from build123d import *

# Parameters (mm, degrees)
SKETCH1_R           = 2.54
BOSS_EXTRUDE1_DEPTH = 3.175
FILLET1_R           = 6.35
FILLET2_R           = 3.175


with BuildPart() as part:
    # Sketch1 → Boss-Extrude1 (new body)
    with BuildSketch(Plane(origin=(0, 0, 0), x_dir=(1, 0, 0), z_dir=(0, 1, 0))):
        Polygon((0, 0), (0, 88.9), (25.4, 88.9), (88.9, 25.4), (88.9, 0), align=None)
        with Locations(Location((12.7, 12.7, 0), (0, 0, 270))):
            Circle(SKETCH1_R, mode=Mode.SUBTRACT)
        with Locations(Location((25.4, 12.7, 0), (0, 0, 270))):
            Circle(SKETCH1_R, mode=Mode.SUBTRACT)
        with Locations(Location((38.1, 12.7, 0), (0, 0, 270))):
            Circle(SKETCH1_R, mode=Mode.SUBTRACT)
        with Locations(Location((50.8, 12.7, 0), (0, 0, 270))):
            Circle(SKETCH1_R, mode=Mode.SUBTRACT)
        with Locations(Location((63.5, 12.7, 0), (0, 0, 270))):
            Circle(SKETCH1_R, mode=Mode.SUBTRACT)
        with Locations(Location((76.2, 12.7, 0), (0, 0, 270))):
            Circle(SKETCH1_R, mode=Mode.SUBTRACT)
        with Locations(Location((12.7, 25.4, 0), (0, 0, 270))):
            Circle(SKETCH1_R, mode=Mode.SUBTRACT)
        with Locations(Location((12.7, 38.1, 0), (0, 0, 270))):
            Circle(SKETCH1_R, mode=Mode.SUBTRACT)
        with Locations(Location((12.7, 50.8, 0), (0, 0, 270))):
            Circle(SKETCH1_R, mode=Mode.SUBTRACT)
        with Locations(Location((12.7, 63.5, 0), (0, 0, 270))):
            Circle(SKETCH1_R, mode=Mode.SUBTRACT)
        with Locations(Location((12.7, 76.2, 0), (0, 0, 270))):
            Circle(SKETCH1_R, mode=Mode.SUBTRACT)
        Polygon((25.4, 25.4), (25.4, 79.919743879), (79.919743879, 25.4), align=None, mode=Mode.SUBTRACT)
    extrude(amount=BOSS_EXTRUDE1_DEPTH)

    # Fillet1
    fillet1_edges = [part.edges().sort_by_distance(p)[0] for p in [
        (0, 1.5875, 0),
        (0, 1.5875, -88.9),
        (25.4, 1.5875, -88.9),
        (88.9, 1.5875, -25.4),
        (88.9, 1.5875, 0),
    ]]
    fillet(fillet1_edges, radius=FILLET1_R)

    # Fillet2
    fillet2_edges = [part.edges().sort_by_distance(p)[0] for p in [
        (25.4, 1.5875, -25.4),
        (79.919743879, 1.5875, -25.4),
        (25.4, 1.5875, -79.919743879),
    ]]
    fillet(fillet2_edges, radius=FILLET2_R)


solid = part.part
Geometry: final body of the model. Coordinates: model frame, mm. A direction names the side the tool comes from. Round coordinates to 2 decimals unless told otherwise and drop trailing zeros. Write each loop counter-clockwise with the first axis right and the second up, starting at its lowest first coordinate (ties: lowest second). Pieces come first, ordered by that corner, then holes. Notation, with made-up numbers: M 17.5,12 L 47.5,12 A13 ccw 47.5,29 Z; hole C 8.5,-25.75 d8. An arc over 180 degrees is marked long. Write item = value, one per line.
Item 1: Section query C-C on y = 2.15. State how many separate pieces and enclosed holes the cut face has, then the cut area to 3 significant figures.
Findings:
separate_pieces = 1
enclosed_holes = 12
area = 4,180 mm^2
Item 2: Section query B-B on x = 12.7. Return loops of the section in (y, z) (3 decimals), then the cut area to 3 significant figures.
Findings:
outline = M 0,-88.9 L 3.175,-88.9 L 3.175,-78.74 L 0,-78.74 Z; M 0,-73.66 L 3.175,-73.66 L 3.175,-66.04 L 0,-66.04 Z; M 0,-60.96 L 3.175,-60.96 L 3.175,-53.34 L 0,-53.34 Z; M 0,-48.26 L 3.175,-48.26 L 3.175,-40.64 L 0,-40.64 Z; M 0,-35.56 L 3.175,-35.56 L 3.175,-27.94 L 0,-27.94 Z; M 0,-22.86 L 3.175,-22.86 L 3.175,-15.24 L 0,-15.24 Z; M 0,-10.16 L 3.175,-10.16 L 3.175,0 L 0,0 Z
area = 185 mm^2
Item 3: Section query A-A on z = -12.7. Return loops of the section in (x, y) (3 decimals), then the cut area to 3 significant figures.
Findings:
outline = M 0,0 L 10.16,0 L 10.16,3.175 L 0,3.175 Z; M 15.24,0 L 22.86,0 L 22.86,3.175 L 15.24,3.175 Z; M 27.94,0 L 35.56,0 L 35.56,3.175 L 27.94,3.175 Z; M 40.64,0 L 48.26,0 L 48.26,3.175 L 40.64,3.175 Z; M 53.34,0 L 60.96,0 L 60.96,3.175 L 53.34,3.175 Z; M 66.04,0 L 73.66,0 L 73.66,3.175 L 66.04,3.175 Z; M 78.74,0 L 88.9,0 L 88.9,3.175 L 78.74,3.175 Z
area = 185 mm^2
Item 4: Pull-direction query (Z, two-part tool) for faces 3 (the face through (25, 0, -35)), 4 (the face through (73.72, 1.57, -13.25)), 5 (the face through (86.99, 1.61, -1.81)); classes: pulls with the +Z half, pulls with the -Z half, needs draft (parallel to the pull), parting line crosses it, or undercut.
Findings:
face_3 = needs draft
face_4 = undercut
face_5 = pulls with the +Z half
Item 5: Material intervals for line 1 along X through (y, z) = (1.45, -37.5); line 2 along X through (y, z) = (1.2, -36); line 3 along X through (y, z) = (0.95, -68), sorted ascending. Write a range as [from, to].
Findings:
line_1 = [0, 10.23], [15.17, 25.4], [67.82, 76.8]
line_2 = [0, 11.27], [14.13, 25.4], [69.32, 78.3]
line_3 = [0, 25.4], [37.32, 46.3]
Item 6: Pin query (flat end, axial travel): P1, Ø6, axis at x = 63.5, z = -12.7, coming from the +Y side (3 decimals); P2, Ø4.5, axis at x = 25.4, z = -12.7, coming from the +Y side; P3, Ø1, axis at y = 2, z = -42.5, coming from the +X side. Return the tip coordinate at first contact, or that it passes through.
Findings:
P1 = 3.175
P2 = through
P3 = 72.3
Item 7: Access query for faces 1 (the face through (27.312, 1.61, -75.167)), 2 (the face through (88.43, 1.61, -25.17)). Directions: +Z, -Z, +X, -X, +Y, -Y. A direction counts if a zero-diameter tool reaches every point of the face in a straight line with its end or side. Return the directions, or none.
Findings:
face_1 = +Y, -Y
face_2 = -Z, +X, +Y, -Y
Item 8: Section query D-D on z = -38.1. Return loops of the section in (x, y) (3 decimals), then the cut area to 3 significant figures.
Findings:
outline = M 0,0 L 10.16,0 L 10.16,3.175 L 0,3.175 Z; M 15.24,0 L 25.4,0 L 25.4,3.175 L 15.24,3.175 Z; M 67.22,0 L 76.2,0 L 76.2,3.175 L 67.22,3.175 Z
area = 93.0 mm^2
